The model under review builds one solid part; all positions refer to its coordinate system, in mm. A direction names the side the tool comes from. Coordinates: 2 decimals unless noted, no trailing zeros. Order: outer loops, then holes, each group sorted by start corner. A loop starts at its lowest first (then second) coordinate and runs counter-clockwise, first axis right, second up. Notation, with made-up numbers: M 40.5,-14.5 L 80.5,-14.5 A15 cw 80.5,-4.5 Z; hole C -23.75,57.25 d11. An arc over 180 degrees is marked long. Write each question's results on one line, items separated by ' | '.
from build123d import *

# Parameters (mm, degrees)
SALIENTE_EXTRUIR1_DEPTH = 170
CROQUIS2_W              = 55
CROQUIS2_H              = 28
CORTAR_EXTRUIR1_DEPTH   = 6
CROQUIS3_W              = 44
CROQUIS3_H              = 60
CORTAR_EXTRUIR2_DEPTH   = 6
CROQUIS4_W              = 4
CROQUIS4_H              = 50
CORTAR_EXTRUIR3_DEPTH   = 10
CROQUIS5_W              = 20.5
CROQUIS5_H              = 12
CROQUIS5_W_2            = 18
CORTAR_EXTRUIR4_DEPTH   = 6
CROQUIS6_W              = 129
CROQUIS6_H              = 16
CORTAR_EXTRUIR5_DEPTH   = 6
CROQUIS7_R              = 5
CORTAR_EXTRUIR6_DEPTH   = 6
REDONDEO1_R             = 5


with BuildPart() as part:
    # Croquis1 → Saliente-Extruir1 (new body)
    with BuildSketch(Plane.XY):
        Polygon((0, 0), (0, 50), (6, 50), (6, 6), (50, 6), (50, 0), align=None)
    extrude(amount=SALIENTE_EXTRUIR1_DEPTH)

    # Croquis2 → Cortar-Extruir1 (cut)
    with BuildSketch(Plane.ZY):
        with Locations((85, 36)):
            Rectangle(CROQUIS2_W, CROQUIS2_H)
        with BuildLine():
            Line((149.5, 35), (149.5, 50))
            Line((149.5, 50), (130.5, 50))
            Line((130.5, 50), (130.5, 35))
            ThreePointArc((130.5, 35), (140, 25.5), (149.5, 35))
        make_face()
        with BuildLine():
            Line((39.5, 35), (39.5, 50))
            Line((39.5, 50), (20.5, 50))
            Line((20.5, 50), (20.5, 35))
            ThreePointArc((20.5, 35), (30, 25.5), (39.5, 35))
        make_face()
    extrude(amount=-CORTAR_EXTRUIR1_DEPTH, mode=Mode.SUBTRACT)

    # Croquis3 → Cortar-Extruir2 (cut)
    with BuildSketch(Plane.XZ):
        with Locations((28, 140)):
            Rectangle(CROQUIS3_W, CROQUIS3_H)
        with Locations((28, 30)):
            Rectangle(CROQUIS3_W, CROQUIS3_H)
    extrude(amount=-CORTAR_EXTRUIR2_DEPTH, mode=Mode.SUBTRACT)

    # Croquis4 → Cortar-Extruir3 (cut)
    with BuildSketch(Plane.XZ):
        with Locations((48, 85)):
            Rectangle(CROQUIS4_W, CROQUIS4_H)
    extrude(amount=-CORTAR_EXTRUIR3_DEPTH, mode=Mode.SUBTRACT)

    # Croquis5 → Cortar-Extruir4 (cut)
    with BuildSketch(Plane.ZY):
        with Locations((159.75, 44)):
            Rectangle(CROQUIS5_W, CROQUIS5_H)
        with Locations((121.5, 44)):
            Rectangle(CROQUIS5_W_2, CROQUIS5_H)
        with Locations((48.5, 44)):
            Rectangle(CROQUIS5_W_2, CROQUIS5_H)
        with Locations((10.25, 44)):
            Rectangle(CROQUIS5_W, CROQUIS5_H)
    extrude(amount=-CORTAR_EXTRUIR4_DEPTH, mode=Mode.SUBTRACT)

    # Croquis6 → Cortar-Extruir5 (cut)
    with BuildSketch(Plane.ZY):
        with Locations((85, 30)):
            Rectangle(CROQUIS6_W, CROQUIS6_H)
    extrude(amount=-CORTAR_EXTRUIR5_DEPTH, mode=Mode.SUBTRACT)

    # Croquis7 → Cortar-Extruir6 (cut)
    with BuildSketch(Plane.XZ):
        with Locations((26, 85)):
            Circle(CROQUIS7_R)
    extrude(amount=-CORTAR_EXTRUIR6_DEPTH, mode=Mode.SUBTRACT)

    # Redondeo1
    redondeo1_edges = [part.edges().sort_by_distance(p)[0] for p in [
        (3, 22, 149.5),
        (3, 22, 20.5),
    ]]
    fillet(redondeo1_edges, radius=REDONDEO1_R)


solid = part.part
1) To check wall thickness, follow line 1 along Z through (x, y) = (26, 4.2); line 2 along Z through (x, y) = (12, 4.5); line 3 along X through (y, z) = (7, 152). State the ranges of each line that lie inside material, in increasing order.
Solutions:
line 1: 60 to 80, 90 to 110 | line 2: 60 to 110 | line 3: 0 to 6
2) For faces 4 (the flat face through (25.7, 6, 90.2)), 5 (the flat face through (26, 3, 110)), 6 (the flat face through (3, 38, 10)), 7 (the flat face through (3, 22, 84)), list the 3-axis set-ups (+Z, -Z, +X, -X, +Y, -Y) from which the entire face can be reached by the end or side of a thin tool; tool diameter is ignored.
Solutions:
face 4: +Z, -Z, +X, +Y | face 5: +Z, +X, +Y, -Y | face 6: +Z, -Z, +X, -X, +Y | face 7: +X, -X, +Y
3) Take a section at B-B on z = 85. State the section outline as (x, y) points, plus the area to 3 significant figures.
Solutions:
outline: M 0,0 L 21,0 L 21,6 L 6,6 L 6,22 L 0,22 Z; M 31,0 L 46,0 L 46,6 L 31,6 Z | area: 312 mm2
4) Take a section at D-D on x = 4. State the section outline as (y, z) points.
Solutions:
outline: M 0,0 L 38,0 L 38,20.5 L 27,20.5 A5 cw 22,25.5 L 22,144.5 A5 cw 27,149.5 L 38,149.5 L 38,170 L 0,170 Z
5) For pin 1 (1.5 mm diameter, centred on y = 11.5, z = 149, fed in from +X); pin 2 (3 mm diameter, centred on x = 27.5, z = 99, fed in from +Y); pin 3 (10 mm diameter, centred on x = 25.5, y = 14, fed in from -Z); pin 4 (1.8 mm diameter, centred on x = 2, y = 33.5, fed in from -Z), all flat-tipped, find the tip position at first contact; note any pin that passes through.
Solutions:
pin 1: x = 6 | pin 2: y = 6 | pin 3: through | pin 4: z = 0
6) The part is to be moulded in two halves that separate along Z. For faces 1 (the cylindrical face through (24.92, 2.96, 80.12)), 2 (the flat face through (6, 15, 84)), 3 (the flat face through (26, 3, 60)), say which applies: pulls with the +Z half, pulls with the -Z half, needs draft (parallel to the pull), parting line crosses it, or undercut.
Solutions:
face 1: undercut | face 2: needs draft | face 3: pulls with the -Z half
7) Take a section at C-C on y = 4. State the section outline as (x, z) points, plus the area to 3 significant figures.
Solutions:
outline: M 0,0 L 6,0 L 6,60 L 46,60 L 46,110 L 6,110 L 6,170 L 0,170 Z; hole C 26,85 d10 | area: 2,940 mm2
8) Take a section at A-A on x = 26. State the section outline as (y, z) points, plus the area to 3 significant figures.
Solutions:
outline: M 0,60 L 6,60 L 6,80 L 0,80 Z; M 0,90 L 6,90 L 6,110 L 0,110 Z | area: 240 mm2
